Verification items for this drawing (mm, ordinates from the low corner). A direction names the side the tool comes from. Coordinates: 2 decimals unless noted, no trailing zeros. Write each loop counter-clockwise with the first axis right and the second up, starting at its lowest first coordinate (ties: lowest second). Pieces come first, ordered by that corner, then holes. Notation, with made-up numbers: (78, -16.5) -> (136, -16.5) arc R32 cw to (136, 16.5) -> close; hole circle Ø3 at (72, 28.25). An arc over 180 degrees is marked (long way). Use CSV: the item, a comma, the result in double quotes.
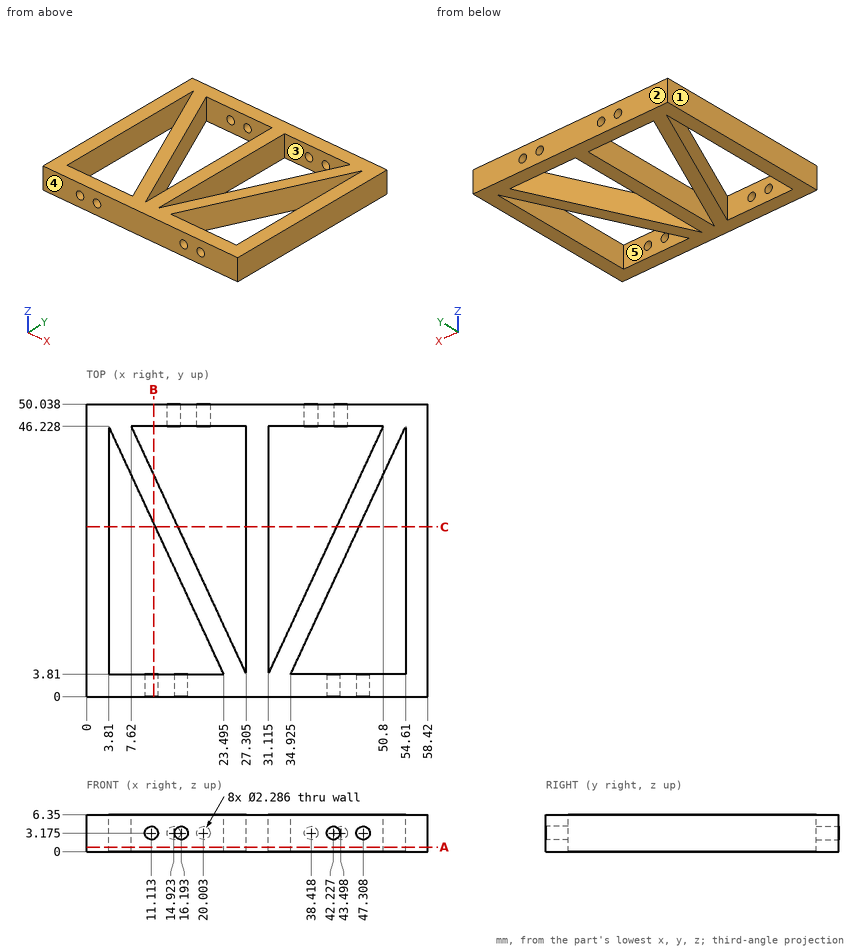
1) Scan lines: L1, parallel to X at y = 22, z = 2.25 (1 decimal); L2, parallel to Y at x = 48.5, z = 1 (1 decimal); L3, parallel to Y at x = 21.5, z = 1.5 (1 decimal). Record each from-to range of solid material in increasing order.
Return value:
L1,"0 to 3.8, 15.1 to 18.9, 27.3 to 31.1, 39.6 to 43.4, 54.6 to 58.4"
L2,"0 to 3.8, 33.1 to 41.3, 46.2 to 50"
L3,"0 to 3.8, 8.1 to 16.3, 46.2 to 50"
2) Set-up check for the marked faces 4 and 5: record each of +Z, -Z, +X, -X, +Y, -Y from which the full face is reachable in a straight line by a thin tool's end or side.
Return value:
face 4,"+Z, -Z, +X, -X, -Y"
face 5,"+Z, -Z"
3) Cross-section at C-C (y = 29). Give the number of separate pieces and of enclosed holes in the cut face, plus the area to 3 significant figures.
Return value:
separate pieces,"5"
enclosed holes,"0"
area,"121 mm2"
4) Mould release check, pull along Y, two halves, no side actions. Record for the marked faces 1, 2 and 3: released by +Y, released by -Y, zero draft, split by the parting line, or undercut.
Return value:
face 1,"zero draft"
face 2,"released by +Y"
face 3,"undercut"
5) Gauge pin test, flat ends, axial feed: pin 1 (1.4 mm diameter, centred on x = 14.92, z = 3.18, fed in from +Y) (1 decimal); pin 2 (2 mm diameter, centred on x = 47.31, z = 3.18, fed in from -Y) (1 decimal). Record the tip position at first contact, or that the pin passes through.
Return value:
pin 1,"y = 32"
pin 2,"y = 28.3"
6) Cross-section at A-A (z = 0.75). Record the boundary of the cut face in (x, y) (1 decimal).
Return value:
outline,"(0, 0) -> (58.4, 0) -> (58.4, 50) -> (0, 50) -> close; hole (3.8, 3.8) -> (23.5, 3.8) -> (3.8, 46.2) -> close; hole (7.6, 46.2) -> (27.3, 3.8) -> (27.3, 46.2) -> close; hole (31.1, 3.8) -> (50.8, 46.2) -> (31.1, 46.2) -> close; hole (34.9, 3.8) -> (54.6, 3.8) -> (54.6, 46.2) -> close"
7) Cross-section at B-B (x = 11.5). Record the boundary of the cut face in (y, z).
Return value:
outline,"(0, 0) -> (3.81, 0) -> (3.81, 2.1) -> (0, 2.1) -> close; (0, 4.25) -> (3.81, 4.25) -> (3.81, 6.35) -> (0, 6.35) -> close; (29.66, 0) -> (37.87, 0) -> (37.87, 6.35) -> (29.66, 6.35) -> close; (46.23, 0) -> (50.04, 0) -> (50.04, 6.35) -> (46.23, 6.35) -> close"
